Part model, mm, in its own coordinate system. Round coordinates to 2 decimals unless told otherwise and drop trailing zeros. Loops run counter-clockwise (first coordinate to the right, second up) from the corner with the lowest first, then second, coordinate; pieces in that order, holes last. Notation, with made-up numbers: (47, 11) - (77, 11) arc R27 cw to (77, 35) - close; hole circle Ø9 at (-36, 42.25). An arc over 180 degrees is marked (long way). Write each question's results on one line, items separated by ' | '. Start each with the question number.
(1) Drill centre lines: L1, parallel to Z at x = 1, y = 2.85; L2, parallel to Z at x = 124.86, y = 2.05; L3, parallel to Z at x = 80, y = 0.5. Where is each one in solid material? Low to high.
(2) Cut at B-B, the plane x = 95. List the corners of the cut face in (y, z).
(3) Cut at A-A, the plane z = -97. List the corners of the cut face in (x, y).
(4) Cut at C-C, the plane y = 1.2. Give the number of separate pieces and of enclosed holes in the cut face, then the cut area to 3 significant figures.
(5) Flat gauge pin, fed straight in: P1, Ø3.5, axis at x = 110, z = -72, coming from the +Y side. Where does the tip first touch, or does it go through?
from build123d import *

# Parameters (mm, degrees)
EXTRUDE_1_DEPTH      = 4
SKETCH_2_R           = 1.5
CUT_EXTRUDE_1_DEPTH  = 4
SKETCH_3_R           = 23.5
SKETCH_3_R_2         = 1.5
CUT_EXTRUDE_2_DEPTH  = 4
SKETCH_4_W           = 90
SKETCH_4_H           = 90
CUT_EXTRUDE_3_DEPTH  = 4
FILLET_3_R           = 6
CHAMFER_1_SIZE       = 10
CUT_EXTRUDE_6_DEPTH  = 4
CHAMFER_2_SIZE       = 15
SKETCH_8_R           = 1.5
CUT_EXTRUDE_7_DEPTH  = 4
SKETCH_9_R           = 1.5
CUT_EXTRUDE_8_DEPTH  = 4
CUT_EXTRUDE_9_DEPTH  = 10
SKETCH_14_R          = 1.5
SKETCH_14_R_2        = 1.25
CUT_EXTRUDE_10_DEPTH = 10
SKETCH_15_R          = 1.5
SKETCH_15_W          = 42
SKETCH_15_H          = 23
CUT_EXTRUDE_11_DEPTH = 10
FILLET_4_R           = 1
SKETCH_16_R          = 1.25
CUT_EXTRUDE_12_DEPTH = 10
SKETCH_23_R          = 1.25
CUT_EXTRUDE_14_DEPTH = 10
SKETCH_24_R          = 1.5
CUT_EXTRUDE_15_DEPTH = 10
SKETCH_20_R          = 1.5
CUT_EXTRUDE_16_DEPTH = 10


with BuildPart() as part:
    # 草图1 → 凸台-拉伸1 (new body)
    with BuildSketch(Plane(origin=(0, 0, 0), x_dir=(1, 0, 0), z_dir=(0, 1, 0))):
        Polygon((-47.5, -81), (-47.5, -135), (47.5, -135), (47.5, -81), (145, -81), (145, 81), (47.5, 81), (47.5, 135), (-47.5, 135), (-47.5, 81), (-145, 81), (-145, -81), align=None)
    extrude(amount=EXTRUDE_1_DEPTH)

    # 草图2 → 切除-拉伸1 (cut)
    with BuildSketch(Plane(origin=(0, 4, 0), x_dir=(1, 0, 0), z_dir=(0, 1, 0))):
        with Locations(Location((110, 72, 0), (0, 0, 270))):
            Circle(SKETCH_2_R)
        with Locations(Location((80, 72, 0), (0, 0, 270))):
            Circle(SKETCH_2_R)
        with Locations(Location((80, 48, 0), (0, 0, 270))):
            Circle(SKETCH_2_R)
        with Locations(Location((110, 48, 0), (0, 0, 270))):
            Circle(SKETCH_2_R)
        with Locations(Location((110, -48, 0), (0, 0, 90))):
            Circle(SKETCH_2_R)
        with Locations(Location((110, -72, 0), (0, 0, 90))):
            Circle(SKETCH_2_R)
        with Locations(Location((80, -48, 0), (0, 0, 90))):
            Circle(SKETCH_2_R)
        with Locations(Location((80, -72, 0), (0, 0, 90))):
            Circle(SKETCH_2_R)
        with Locations(Location((-80, -72, 0), (0, 0, 270))):
            Circle(SKETCH_2_R)
        with Locations(Location((-80, -48, 0), (0, 0, 270))):
            Circle(SKETCH_2_R)
        with Locations(Location((-110, -72, 0), (0, 0, 270))):
            Circle(SKETCH_2_R)
        with Locations(Location((-110, -48, 0), (0, 0, 270))):
            Circle(SKETCH_2_R)
        with Locations(Location((-110, 48, 0), (0, 0, 90))):
            Circle(SKETCH_2_R)
        with Locations(Location((-80, 48, 0), (0, 0, 90))):
            Circle(SKETCH_2_R)
        with Locations(Location((-80, 72, 0), (0, 0, 90))):
            Circle(SKETCH_2_R)
        with Locations(Location((-110, 72, 0), (0, 0, 90))):
            Circle(SKETCH_2_R)
    extrude(amount=-CUT_EXTRUDE_1_DEPTH, mode=Mode.SUBTRACT)

    # 草图3 → 切除-拉伸2 (cut)
    with BuildSketch(Plane(origin=(0, 4, 0), x_dir=(1, 0, 0), z_dir=(0, 1, 0))):
        with Locations(Location((0, 97, 0), (0, 0, 270))):
            Circle(SKETCH_3_R)
        with Locations(Location((29, 122, 0), (0, 0, 270))):
            Circle(SKETCH_3_R_2)
        with Locations(Location((29, 72, 0), (0, 0, 90))):
            Circle(SKETCH_3_R_2)
        with Locations(Location((-29, 72, 0), (0, 0, 270))):
            Circle(SKETCH_3_R_2)
        with Locations(Location((-29, 122, 0), (0, 0, 90))):
            Circle(SKETCH_3_R_2)
    extrude(amount=-CUT_EXTRUDE_2_DEPTH, mode=Mode.SUBTRACT)

    # 草图4 → 切除-拉伸3 (cut)
    with BuildSketch(Plane(origin=(0, 4, 0), x_dir=(1, 0, 0), z_dir=(0, 1, 0))):
        Rectangle(SKETCH_4_W, SKETCH_4_H)
    extrude(amount=-CUT_EXTRUDE_3_DEPTH, mode=Mode.SUBTRACT)

    # 圆角3
    fillet_3_edges = [part.edges().sort_by_distance(p)[0] for p in [
        (-145, 2, 81),
        (-145, 2, -81),
        (-47.5, 2, -135),
        (47.5, 2, -135),
        (145, 2, -81),
        (145, 2, 81),
        (47.5, 2, 135),
        (-47.5, 2, 135),
    ]]
    fillet(fillet_3_edges, radius=FILLET_3_R)

    # 倒角1
    chamfer_1_edges = [part.edges().sort_by_distance(p)[0] for p in [
        (-47.5, 2, 81),
        (-47.5, 2, -81),
        (47.5, 2, -81),
        (47.5, 2, 81),
    ]]
    chamfer(chamfer_1_edges, length=CHAMFER_1_SIZE)

    # 草图7 → 切除-拉伸6 (cut)
    with BuildSketch(Plane(origin=(0, 4, 0), x_dir=(1, 0, 0), z_dir=(0, 1, 0))):
        with BuildLine():
            Line((-65, -20), (-65, 20))
            ThreePointArc((-65, 20), (-58, 27), (-51, 20))
            Line((-51, 20), (-51, -20))
            ThreePointArc((-51, -20), (-58, -27), (-65, -20))
        make_face()
        with BuildLine():
            Line((-141, -15), (-141, 15))
            ThreePointArc((-141, 15), (-137, 19), (-133, 15))
            Line((-133, 15), (-133, -15))
            ThreePointArc((-133, -15), (-137, -19), (-141, -15))
        make_face()
        with BuildLine():
            Line((129, 38), (129, 52))
            ThreePointArc((129, 52), (134, 57), (139, 52))
            Line((139, 52), (139, 38))
            ThreePointArc((139, 38), (134, 33), (129, 38))
        make_face()
        with BuildLine():
            Line((129, -38), (129, -52))
            ThreePointArc((129, -52), (134, -57), (139, -52))
            Line((139, -52), (139, -38))
            ThreePointArc((139, -38), (134, -33), (129, -38))
        make_face()
    extrude(amount=-CUT_EXTRUDE_6_DEPTH, mode=Mode.SUBTRACT)

    # 倒角2
    chamfer_2_edges = [part.edges().sort_by_distance(p)[0] for p in [
        (45, 2, -45),
        (45, 2, 45),
        (-45, 2, 45),
        (-45, 2, -45),
    ]]
    chamfer(chamfer_2_edges, length=CHAMFER_2_SIZE)

    # 草图8 → 切除-拉伸7 (cut)
    with BuildSketch(Plane(origin=(0, 4, 0), x_dir=(1, 0, 0), z_dir=(0, 1, 0))):
        with Locations(Location((-139, 60, 0), (0, 0, 270))):
            Circle(SKETCH_8_R)
        with Locations(Location((-131, 60, 0), (0, 0, 270))):
            Circle(SKETCH_8_R)
    extrude(amount=-CUT_EXTRUDE_7_DEPTH, mode=Mode.SUBTRACT)

    # 草图9 → 切除-拉伸8 (cut)
    with BuildSketch(Plane(origin=(0, 4, 0), x_dir=(1, 0, 0), z_dir=(0, 1, 0))):
        with Locations(Location((50.843145751, 56.5, 0), (0, 0, 270))):
            Circle(SKETCH_9_R)
        with Locations(Location((56.5, 50.843145751, 0), (0, 0, 270))):
            Circle(SKETCH_9_R)
        with Locations(Location((56.5, -50.843145751, 0), (0, 0, 90))):
            Circle(SKETCH_9_R)
        with Locations(Location((50.843145751, -56.5, 0), (0, 0, 90))):
            Circle(SKETCH_9_R)
        with Locations(Location((-50.843145751, -56.5, 0), (0, 0, 270))):
            Circle(SKETCH_9_R)
        with Locations(Location((-56.5, -50.843145751, 0), (0, 0, 270))):
            Circle(SKETCH_9_R)
        with Locations(Location((-56.5, 50.843145751, 0), (0, 0, 90))):
            Circle(SKETCH_9_R)
        with Locations(Location((-50.843145751, 56.5, 0), (0, 0, 90))):
            Circle(SKETCH_9_R)
        with Locations(Location((-37.5, -127, 0), (0, 0, 270))):
            Circle(SKETCH_9_R)
        with Locations(Location((37.5, -127, 0), (0, 0, 90))):
            Circle(SKETCH_9_R)
    extrude(amount=-CUT_EXTRUDE_8_DEPTH, mode=Mode.SUBTRACT)

    # 草图12 → 切除-拉伸9 (cut)
    with BuildSketch(Plane(origin=(0, 4, 0), x_dir=(1, 0, 0), z_dir=(0, 1, 0))):
        with BuildLine():
            Line((-20, -54), (20, -54))
            ThreePointArc((20, -54), (26, -60), (20, -66))
            Line((20, -66), (-20, -66))
            ThreePointArc((-20, -66), (-26, -60), (-20, -54))
        make_face()
    extrude(amount=-CUT_EXTRUDE_9_DEPTH, mode=Mode.SUBTRACT)

    # 草图14 → 切除-拉伸10 (cut)
    with BuildSketch(Plane(origin=(0, 4, 0), x_dir=(1, 0, 0), z_dir=(0, 1, 0))):
        with Locations(Location((36, -79, 0), (0, 0, 270))):
            Circle(SKETCH_14_R)
        with Locations(Location((36, -121, 0), (0, 0, 270))):
            Circle(SKETCH_14_R)
        with Locations(Location((-36, -121, 0), (0, 0, 270))):
            Circle(SKETCH_14_R)
        with Locations(Location((-36, -79, 0), (0, 0, 270))):
            Circle(SKETCH_14_R)
        with Locations(Location((-24.5, -71, 0), (0, 0, 270))):
            Circle(SKETCH_14_R_2)
        with Locations(Location((24.5, -71, 0), (0, 0, 270))):
            Circle(SKETCH_14_R_2)
        with Locations(Location((24.5, -129, 0), (0, 0, 270))):
            Circle(SKETCH_14_R_2)
        with Locations(Location((-24.5, -129, 0), (0, 0, 270))):
            Circle(SKETCH_14_R_2)
    extrude(amount=-CUT_EXTRUDE_10_DEPTH, mode=Mode.SUBTRACT)

    # 草图15 → 切除-拉伸11 (cut)
    with BuildSketch(Plane(origin=(0, 4, 0), x_dir=(1, 0, 0), z_dir=(0, 1, 0))):
        with Locations(Location((75.36, 5, 0), (0, 0, 270))):
            Circle(SKETCH_15_R)
        with Locations(Location((75.36, -5, 0), (0, 0, 270))):
            Circle(SKETCH_15_R)
        with Locations(Location((124.86, -5, 0), (0, 0, 270))):
            Circle(SKETCH_15_R)
        with Locations(Location((124.86, 5, 0), (0, 0, 270))):
            Circle(SKETCH_15_R)
        with Locations((100.11, 0)):
            Rectangle(SKETCH_15_W, SKETCH_15_H)
    extrude(amount=-CUT_EXTRUDE_11_DEPTH, mode=Mode.SUBTRACT)

    # 圆角4
    fillet_4_edges = [part.edges().sort_by_distance(p)[0] for p in [
        (121.11, 2, -11.5),
        (121.11, 2, 11.5),
        (79.11, 2, 11.5),
        (79.11, 2, -11.5),
    ]]
    fillet(fillet_4_edges, radius=FILLET_4_R)

    # 草图16 → 切除-拉伸12 (cut)
    with BuildSketch(Plane(origin=(0, 4, 0), x_dir=(1, 0, 0), z_dir=(0, 1, 0))):
        with Locations(Location((-73.5, 41, 0), (0, 0, 270))):
            Circle(SKETCH_16_R)
        with Locations(Location((-122.5, 41, 0), (0, 0, 270))):
            Circle(SKETCH_16_R)
        with Locations(Location((-73.5, -17, 0), (0, 0, 270))):
            Circle(SKETCH_16_R)
        with Locations(Location((-122.5, -17, 0), (0, 0, 270))):
            Circle(SKETCH_16_R)
    extrude(amount=-CUT_EXTRUDE_12_DEPTH, mode=Mode.SUBTRACT)

    # 草图23 → 切除-拉伸14 (cut)
    with BuildSketch(Plane(origin=(0, 4, 0), x_dir=(1, 0, 0), z_dir=(0, 1, 0))):
        with Locations(Location((-81, 31, 0), (0, 0, 270))):
            Circle(SKETCH_23_R)
        with Locations(Location((-139, 31, 0), (0, 0, 270))):
            Circle(SKETCH_23_R)
        with Locations(Location((-81, -55, 0), (0, 0, 270))):
            Circle(SKETCH_23_R)
        with Locations(Location((-139, -55, 0), (0, 0, 270))):
            Circle(SKETCH_23_R)
    extrude(amount=-CUT_EXTRUDE_14_DEPTH, mode=Mode.SUBTRACT)

    # 草图24 → 切除-拉伸15 (cut)
    with BuildSketch(Plane(origin=(0, 4, 0), x_dir=(1, 0, 0), z_dir=(0, 1, 0))):
        with Locations(Location((-136, -71, 0), (0, 0, 270))):
            Circle(SKETCH_24_R)
        with Locations(Location((-36, -71, 0), (0, 0, 270))):
            Circle(SKETCH_24_R)
        with Locations(Location((-36, -121, 0), (0, 0, 270))):
            Circle(SKETCH_24_R)
    extrude(amount=-CUT_EXTRUDE_15_DEPTH, mode=Mode.SUBTRACT)

    # 草图20 → 切除-拉伸16 (cut)
    with BuildSketch(Plane(origin=(0, 4, 0), x_dir=(1, 0, 0), z_dir=(0, 1, 0))):
        with Locations(Location((-60, 60, 0), (0, 0, 270))):
            Circle(SKETCH_20_R)
    extrude(amount=-CUT_EXTRUDE_16_DEPTH, mode=Mode.SUBTRACT)


solid = part.part
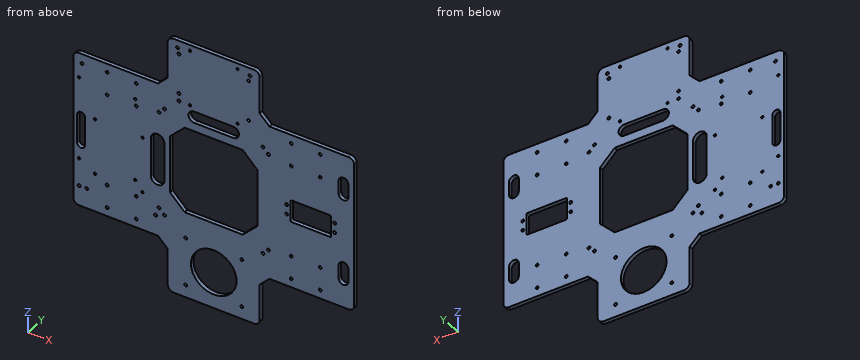
A:
1) L1: -135 to -120.48, -73.52 to -45, 45 to 54, 66 to 135 | L2: -81 to -6.5, -3.5 to 3.5, 6.5 to 81 | L3: -81 to -73.5, -70.5 to -49.5, -46.5 to -11.49, 11.49 to 46.5, 49.5 to 70.5, 73.5 to 81
2) outline: (0, -81) - (4, -81) - (4, -11.5) - (0, -11.5) - close; (0, 11.5) - (4, 11.5) - (4, 81) - (0, 81) - close
3) outline: (-47.5, 0) - (-23.5, 0) - (-23.5, 4) - (-47.5, 4) - close; (23.5, 0) - (47.5, 0) - (47.5, 4) - (23.5, 4) - close
4) separate pieces: 1 | enclosed holes: 63 | area: 44,600 mm2
5) P1: y = 4
